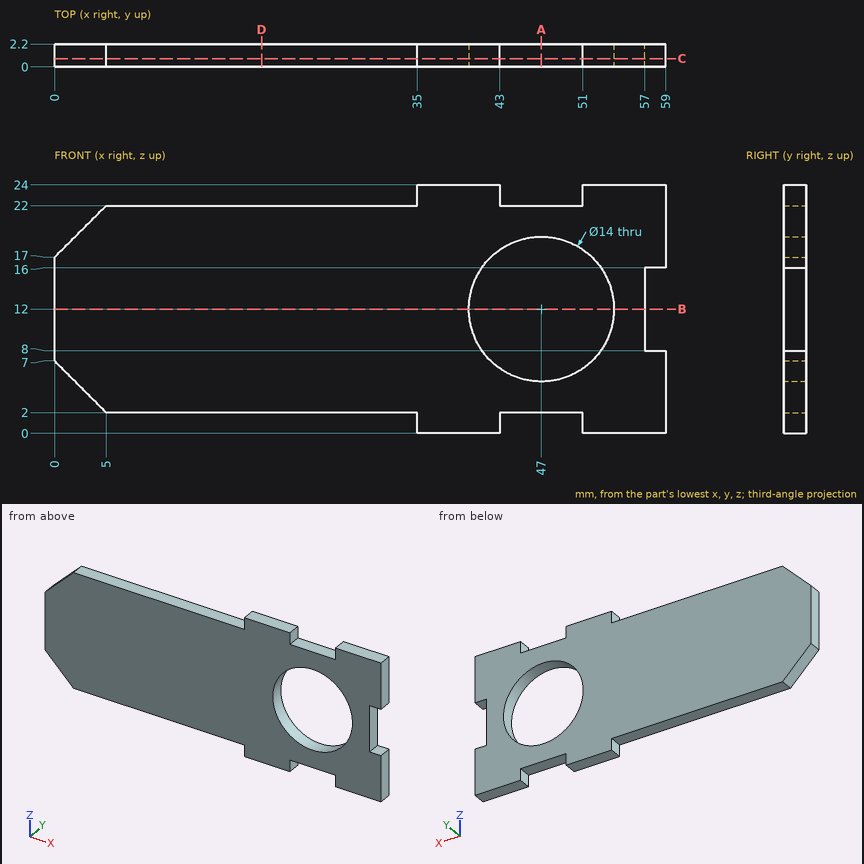
Job drawing, mm, ordinate dimensions from the low corner. One solid piece. Round coordinates to 2 decimals unless told otherwise and drop trailing zeros. Loops run counter-clockwise (first coordinate to the right, second up) from the corner with the lowest first, then second, coordinate; pieces in that order, holes last.
(1) Cut at C-C (y = 0.8). Give the cut face in (x, z), plus the area to 3 significant figures.
(2) Cut at A-A (x = 47). Give the cut face in (y, z).
(3) Cut at B-B (z = 12). Give the cut face in (x, y), plus the area to 3 significant figures.
(4) Cut at D-D (x = 20). Give the cut face in (y, z), plus the area to 3 significant figures.
(5) Drop flat-ended pins along their axis: pin 1 (8 mm diameter, centred on x = 7.5, z = 4, fed in from -Y); pin 2 (0.6 mm diameter, centred on y = 1, z = 23, fed in from -X); pin 3 (1 mm diameter, centred on x = 11, y = 1, fed in from +Z). Give the stop position or say it passes through.
(6) Wall check: line 1 along X through (y, z) = (1, 12); line 2 along X through (y, z) = (1.55, 1.5); line 3 along Z through (x, y) = (25, 1.4). Give the ranges that are in metal, low to high.
Findings below:
1. outline: (0, 7) - (5, 2) - (35, 2) - (35, 0) - (43, 0) - (43, 2) - (51, 2) - (51, 0) - (59, 0) - (59, 8) - (57, 8) - (57, 16) - (59, 16) - (59, 24) - (51, 24) - (51, 22) - (43, 22) - (43, 24) - (35, 24) - (35, 22) - (5, 22) - (0, 17) - close; hole circle Ø14 at (47, 12)
1. area: 1,050 mm2
2. outline: (0, 2) - (2.2, 2) - (2.2, 5) - (0, 5) - close; (0, 19) - (2.2, 19) - (2.2, 22) - (0, 22) - close
3. outline: (0, 0) - (40, 0) - (40, 2.2) - (0, 2.2) - close; (54, 0) - (57, 0) - (57, 2.2) - (54, 2.2) - close
3. area: 94.6 mm2
4. outline: (0, 2) - (2.2, 2) - (2.2, 22) - (0, 22) - close
4. area: 44.0 mm2
5. pin 1: stops at y = 0
5. pin 2: stops at x = 35
5. pin 3: stops at z = 22
6. line 1: x = 0 to 40, 54 to 57
6. line 2: x = 35 to 43, 51 to 59
6. line 3: z = 2 to 22
